Design review of the part shown in the three views and the two pictorial views. Dimensions are in mm from the part's minimum x, y and z. A direction names the side the tool comes from. Coordinates: 2 decimals unless noted, no trailing zeros. Write each loop counter-clockwise with the first axis right and the second up, starting at its lowest first coordinate (ties: lowest second). Pieces come first, ordered by that corner, then holes. Notation, with made-up numbers: (-5, -21) -> (0, -21) arc R17 cw to (0, -12) -> close; hole circle Ø7 at (63.5, 56.5). An arc over 180 degrees is marked (long way). Answer in a Markdown table with one row per item. Add a question column.
Item 1: For the marked faces 1 and 2, list the 3-axis set-ups (+Z, -Z, +X, -X, +Y, -Y) from which the entire face can be reached by the end or side of a thin tool; tool diameter is ignored.
Item 2: To check wall thickness, follow line 1 (Z direction, x = 6, y = 4.75); line 2 (Y direction, x = 3.25, z = 14) (3 decimals); line 3 (X direction, y = 4.25, z = 17) (1 decimal). State the ranges of each line that lie inside material, in increasing order.
Item 3: Clearance check with a flat-ended pin moving along its axis: P1, Ø2, axis at y = 3.5, z = 7.5, coming from the -X side (3 decimals). State where the tip first meets the part, or that it passes through.
Item 4: Take a section at B-B, the plane x = 5. Write out the cut boundary in (y, z).
Item 5: Take a section at C-C, the plane y = 0.5. Write out the cut boundary in (x, z).
Item 6: Take a section at A-A, the plane z = 29. Write out the cut boundary in (x, y) (3 decimals).
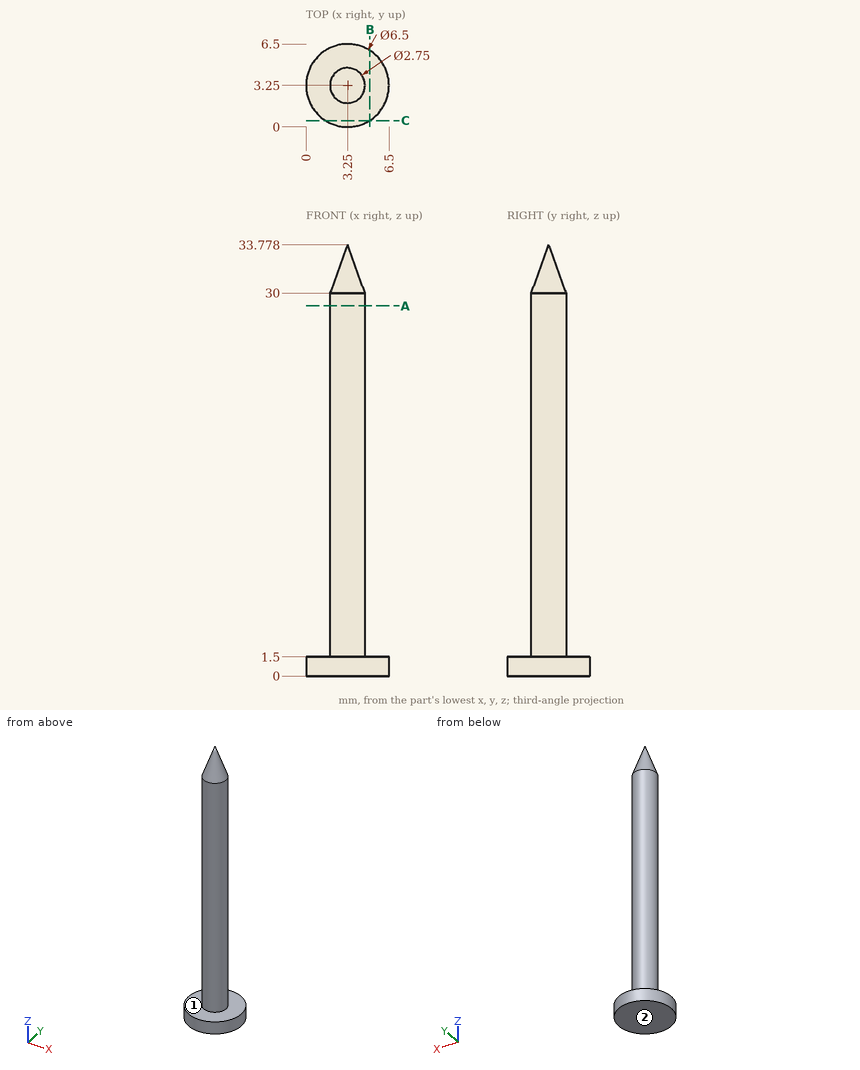
Answers:
| question | item | result |
|---|---|---|
| 1 | face 1 | +Z |
| 1 | face 2 | -Z, +X, -X, +Y, -Y |
| 2 | line 1 | z = 0 to 1.5 |
| 2 | line 2 | y = 1.875 to 4.625 |
| 2 | line 3 | x = 2.3 to 4.2 |
| 3 | P1 | stops at x = 1.875 |
| 4 | outline | (0.51, 0) -> (5.99, 0) -> (5.99, 1.5) -> (0.51, 1.5) -> close |
| 5 | outline | (1.52, 0) -> (4.98, 0) -> (4.98, 1.5) -> (1.52, 1.5) -> close |
| 6 | outline | circle Ø2.75 at (3.25, 3.25) |
